```python
from build123d import *

# Parameters (mm, degrees)
SKETCH1_W           = 19.2
SKETCH1_H           = 33.566975924
BOSS_EXTRUDE1_DEPTH = 5
FILLET1_R           = 2
SKETCH2_W           = 19.2
SKETCH2_H           = 10
CUT_EXTRUDE1_DEPTH  = 0.5
FILLET2_R           = 0.5
CHAMFER1_SIZE       = 0.5


with BuildPart() as part:
    # Sketch1 → Boss-Extrude1 (new body)
    with BuildSketch(Plane.XY):
        with Locations((0, -16.783487962)):
            Rectangle(SKETCH1_W, SKETCH1_H)
        with BuildLine():
            Line((-1.7, -28.866975924), (-1.7, -17.750874329))
            ThreePointArc((-1.7, -17.750874329), (0, -16.050874329), (1.7, -17.750874329))
            Line((1.7, -17.750874329), (1.7, -28.866975924))
            ThreePointArc((1.7, -28.866975924), (0, -30.566975924), (-1.7, -28.866975924))
        make_face(mode=Mode.SUBTRACT)
    extrude(amount=BOSS_EXTRUDE1_DEPTH)

    # Fillet1
    fillet1_edges = [part.edges().sort_by_distance(p)[0] for p in [
        (-9.6, -33.566975924, 2.5),
        (9.6, -33.566975924, 2.5),
    ]]
    fillet(fillet1_edges, radius=FILLET1_R)

    # Sketch2 → Cut-Extrude1 (cut)
    with BuildSketch(Plane.XY):
        with Locations((0, -5)):
            Rectangle(SKETCH2_W, SKETCH2_H)
    extrude(amount=CUT_EXTRUDE1_DEPTH, mode=Mode.SUBTRACT)

    # Fillet2
    fillet2_edges = [part.edges().sort_by_distance(p)[0] for p in [
        (-9.6, 0, 2.75),
        (9.6, 0, 2.75),
    ]]
    fillet(fillet2_edges, radius=FILLET2_R)

    # Chamfer1
    chamfer1_edges = [part.edges().sort_by_distance(p)[0] for p in [
        (-9.6, -20.783487962, 0),
        (-9.014213562, -32.981189486, 0),
        (0, -33.566975924, 0),
        (9.014213562, -32.981189486, 0),
        (9.6, -20.783487962, 0),
    ]]
    chamfer(chamfer1_edges, length=CHAMFER1_SIZE)


solid = part.part
```
Can you work these out from the model? Positions are in its coordinate system, mm. A direction names the side the tool comes from. Give positions to 0.01 mm unless a question says otherwise; leave off trailing zeros. Write each loop counter-clockwise with the first axis right and the second up, starting at its lowest first coordinate (ties: lowest second). Pieces come first, ordered by that corner, then holes. Notation, with made-up numbers: (-25, -20) -> (3, -20) arc R20 cw to (3, 7) -> close; hole circle Ø11 at (4, -28). An arc over 180 degrees is marked (long way). Write item = value, one per line.
(1) Suppose I cut it at A-A on x = 0. Write out the boundary of the cut face in (y, z).
Worked out:
outline = (-33.57, 0.5) -> (-33.07, 0) -> (-30.57, 0) -> (-30.57, 5) -> (-33.57, 5) -> close; (-16.05, 0) -> (-10, 0) -> (-10, 0.5) -> (0, 0.5) -> (0, 5) -> (-16.05, 5) -> close
(2) For faces 5 (the face through (0, -5, 0.5)), 6 (the face through (0, 0, 3)), 7 (the face through (0.037, -30.567, 2.465)), which set-ups out of +Z, -Z, +X, -X, +Y, -Y let a thin tool reach every point of the face, with its end or its side?
Worked out:
face_5 = -Z, +X, -X, +Y
face_6 = +Z, -Z, +X, -X, +Y
face_7 = +Z, -Z
(3) Thinking about a two-plate mould opening in Y: for faces 1 (the face through (-1.7, -23, 2)), 2 (the face through (1.7, -23, 2)), 3 (the face through (8.769, -32.711, 0.135)), 4 (the face through (-9.6, -16, 3)), which applies, released by +Y, released by -Y, zero draft, split by the parting line, or undercut?
Worked out:
face_1 = undercut
face_2 = undercut
face_3 = released by -Y
face_4 = zero draft
(4) Suppose I cut it at D-D on x = -6. Write out the boundary of the cut face in (y, z), then the cut area to 3 significant figures.
Worked out:
outline = (-33.57, 0.5) -> (-33.07, 0) -> (-10, 0) -> (-10, 0.5) -> (0, 0.5) -> (0, 5) -> (-33.57, 5) -> close
area = 163 mm^2
(5) Suppose I cut it at C-C on y = -23. Write out the boundary of the cut face in (x, z), then the cut area to 4 significant figures.
Worked out:
outline = (-9.6, 0.5) -> (-9.1, 0) -> (-1.7, 0) -> (-1.7, 5) -> (-9.6, 5) -> close; (1.7, 0) -> (9.1, 0) -> (9.6, 0.5) -> (9.6, 5) -> (1.7, 5) -> close
area = 78.75 mm^2
(6) I'm going to push a flat-ended pin straight in: P1, Ø8, axis at x = 0.5, y = -3, coming from the -Z side. Where does the tip first touch, or does it pass through?
Worked out:
P1 = 0.5
(7) Suppose I cut it at B-B on z = 2.3. Write out the boundary of the cut face in (x, y).
Worked out:
outline = (-9.6, -31.57) arc R2 ccw to (-7.6, -33.57) -> (7.6, -33.57) arc R2 ccw to (9.6, -31.57) -> (9.6, -0.5) arc R0.5 ccw to (9.1, 0) -> (-9.1, 0) arc R0.5 ccw to (-9.6, -0.5) -> close; hole (-1.7, -28.87) arc R1.7 ccw to (1.7, -28.87) -> (1.7, -17.75) arc R1.7 ccw to (-1.7, -17.75) -> close
(8) I need wall thicknesses on probe 1 along X at (y, z) = (-24, 0.7); probe 2 along Z at (x, y) = (4, -1.5); probe 3 along Y at (x, z) = (1.25, 2). Which ranges of each line are inside material? Lowest first, please. Write a range as from..to.
Worked out:
probe_1 = -9.6..-1.7, 1.7..9.6
probe_2 = 0.5..5
probe_3 = -33.57..-30.02, -16.6..0
